from build123d import *

# Parameters (mm, degrees)
SKETCH1_W           = 76.2
SKETCH1_H           = 584.2
SKETCH1_R           = 12.7
BOSS_EXTRUDE1_DEPTH = 3
SKETCH2_W           = 76.2
SKETCH2_H           = 28.777191139
CUT_OUT_DEPTH       = 586.4487595


with BuildPart() as part:
    # Sketch1 → Boss-Extrude1 (new body)
    with BuildSketch(Plane.XY):
        with Locations((0, 292.1)):
            Rectangle(SKETCH1_W, SKETCH1_H)
        with Locations((0, 555.422808861)):
            Circle(SKETCH1_R, mode=Mode.SUBTRACT)
    extrude(amount=BOSS_EXTRUDE1_DEPTH)

    # Sketch2 → Cut Out (cut, through all)
    with BuildSketch(Plane.XY.offset(3)):
        with Locations((0, 569.811404431)):
            Rectangle(SKETCH2_W, SKETCH2_H)
    extrude(amount=-CUT_OUT_DEPTH, mode=Mode.SUBTRACT)


solid = part.part
The model under review builds one solid part; all positions refer to its coordinate system, in mm. Coordinates: 2 decimals unless noted, no trailing zeros. Write each loop counter-clockwise with the first axis right and the second up, starting at its lowest first coordinate (ties: lowest second). Pieces come first, ordered by that corner, then holes. Notation, with made-up numbers: (-36, 83.5) -> (-6, 83.5) arc R20 cw to (-6, 106.5) -> close; hole circle Ø8 at (-12, 21). An arc over 180 degrees is marked (long way). Answer in a Markdown table with one row per item.
1. Wall thickness on probe 1 along Y at (x, z) = (7, 0.45); probe 2 along Y at (x, z) = (-10, 1.05): over which ranges is each line inside the solid? List them lowest first. Write a range as [from, to].
Answers below:
| item | result |
|---|---|
| probe 1 | y = [0, 544.83] |
| probe 2 | y = [0, 547.59] |
2. We need section A-A, the plane x = 0. State the section outline as (y, z) points.
Answers below:
| item | result |
|---|---|
| outline | (0, 0) -> (542.72, 0) -> (542.72, 3) -> (0, 3) -> close |
3. Draft analysis for pull direction X (two halves, no side actions). For faces 1 (the flat face through (-1, 282, 3)), 2 (the cylindrical face through (-0.279, 542.726, 1.479)), state which applies: +X half, -X half, draft (parallel to the pull), parting line (faces both ways), or undercut.
Answers below:
| item | result |
|---|---|
| face 1 | draft |
| face 2 | undercut |
